Build history of the part. All positions in model axes, mm. A direction names the side the tool comes from. Give positions to 0.01 mm unless a question says otherwise; leave off trailing zeros. Order: outer loops, then holes, each group sorted by start corner. A loop starts at its lowest first (then second) coordinate and runs counter-clockwise, first axis right, second up. Notation, with made-up numbers: (1, -25.5) - (44, -25.5) arc R17 ccw to (44, -18.5) - close; hole circle Ø2 at (36.25, 11). An arc over 180 degrees is marked (long way). Use a Markdown table: item, result. Add a question column.
(1) Flat gauge pins, fed straight in: pin 1 (8 mm diameter, centred on x = 4, z = -31.5, fed in from -Y); pin 2 (8 mm diameter, centred on y = 38, z = 5.5, fed in from +X); pin 3 (5 mm diameter, centred on x = 7, y = 14, fed in from +Z). Where does each tip first touch, or does it go through?
(2) Mould opens along Z. For faces 5 (the face through (0, 39, 19)), 6 (the face through (-0.13, 35.9, 10.98)), 7 (the face through (0, 37, -198)), 8 (the face through (9, 41, 7)) say: +Z half, -Z half, draft (parallel to the pull), parting line (faces both ways), or undercut.
(3) Slice it at A-A (z = -42). Write the cut outline in (x, y).
(4) Slice it at D-D (x = -13.5). Write the cut outline in (y, z).
(5) Slice it at C-C (y = 14.5). Write the cut outline in (x, z), then the cut area to 3 significant figures.
(6) Slice it at B-B (z = 2). Write the cut outline in (x, y).
(7) Wall check: line 1 (Z direction, x = 0, y = 39); line 2 (Y direction, x = 0, z = -66.5); line 3 (Z direction, x = -6, y = 36). Give the ranges that are in metal, low to high.
(8) Which spindle directions (+Z, -Z, +X, -X, +Y, -Y) get a long thin tool onto all of the face, cutting with end or side? Do faces 1 (the face through (-9.237, 32.63, -188.367)), 2 (the face through (-13.047, 50.472, -97.88)), 3 (the face through (-7.797, 31.141, 9.633)), 4 (the face through (0, 48, 9)). Say none if no direction does.
from build123d import *

# Parameters (mm, degrees)
SKETCH_1_R               = 20
EXTRUDE_1_DEPTH          = 19
SKETCH_2_R               = 17
SKETCH_2_R_2             = 10
EXTRUDE_2_DEPTH          = 160
EXTRUDE_START            = 160
SKETCH_2_3_R             = 10
EXTRUDE_3_DEPTH          = 19
CUT_EXTRUDE_1_DEPTH      = 208.569265548
CUT_EXTRUDE_1_DEPTH_BACK = 208.569265548
SKETCH_3_R               = 3.25
SKETCH_4_R               = 19
EXTRUDE_4_DEPTH          = 75
SKETCH_5_W               = 18
SKETCH_5_H               = 18
EXTRUDE_5_DEPTH          = 19
FILLET_1_R               = 4
SKETCH_6_R               = 3.25
CUT_EXTRUDE_2_DEPTH      = 209.628857159


with BuildPart() as part:
    # Sketch 1 → Extrude 1 (new body)
    with BuildSketch(Plane.XY):
        with BuildLine():
            Line((-20, 49), (-20, 0))
            ThreePointArc((-20, 0), (0, 20), (20, 0))
            Line((20, 0), (20, 49))
            Line((20, 49), (10, 59))
            Line((10, 59), (-10, 59))
            Line((-10, 59), (-20, 49))
        make_face()
        Circle(SKETCH_1_R)
    extrude(amount=-EXTRUDE_1_DEPTH)

    # Sketch 2 → Extrude 2 (add)
    # profile 1 of 3: a face of its own
    with BuildSketch(Plane(origin=(0, 0, -19), x_dir=(-1, 0, 0), z_dir=(0, 0, -1))):
        with BuildLine():
            Line((10, 59), (-10, 59))
            Line((-10, 59), (-16.009113575, 42.179115539))
            ThreePointArc((-16.009113575, 42.179115539), (0, 53.46), (16.009113575, 42.179115539))
            Line((16.009113575, 42.179115539), (10, 59))
        make_face()
    # profile 2 of 3: a face of its own
    with BuildSketch(Plane(origin=(0, 0, -19), x_dir=(-1, 0, 0), z_dir=(0, 0, -1))):
        with Locations((0, 36.46)):
            Circle(SKETCH_2_R)
        with Locations((0, 36.46)):
            Circle(SKETCH_2_R_2, mode=Mode.SUBTRACT)
    # profile 3 of 3: a face of its own
    with BuildSketch(Plane(origin=(0, 0, -19), x_dir=(-1, 0, 0), z_dir=(0, 0, -1))):
        with Locations((0, 36.46)):
            Circle(SKETCH_2_R_2)
    extrude(amount=EXTRUDE_2_DEPTH)

    # Sketch 2_3 → Extrude 3 (add)
    with BuildSketch(Plane(origin=(0, 0, -19), x_dir=(-1, 0, 0), z_dir=(0, 0, -1)).offset(EXTRUDE_START)):
        with Locations((0, 36.46)):
            Circle(SKETCH_2_3_R)
    extrude(amount=EXTRUDE_3_DEPTH)

    # Sketch 3 → Cut-Extrude 1 (cut, two sides: drawn at the far end of the back side and taken through both)
    with BuildSketch(Plane(origin=(0, 0, 0), x_dir=(0, 0, -1), z_dir=(1, 0, 0)).offset(-CUT_EXTRUDE_1_DEPTH_BACK)):
        with Locations((189, 36)):
            Circle(SKETCH_3_R)
    extrude(amount=CUT_EXTRUDE_1_DEPTH + CUT_EXTRUDE_1_DEPTH_BACK, mode=Mode.SUBTRACT)

    # Sketch 4 → Extrude 4 (add)
    with BuildSketch(Plane(origin=(0, 0, -19), x_dir=(-1, 0, 0), z_dir=(0, 0, -1))):
        with Locations(Location((0, 0, 0), (0, 0, 180))):
            Circle(SKETCH_4_R)
    extrude(amount=EXTRUDE_4_DEPTH)

    # Sketch 5 → Extrude 5 (add)
    with BuildSketch(Plane.XY):
        with Locations((0, 39)):
            Rectangle(SKETCH_5_W, SKETCH_5_H)
    extrude(amount=EXTRUDE_5_DEPTH)

    # Fillet 1
    fillet_1_edges = [part.edges().sort_by_distance(p)[0] for p in [
        (9, 30, 9.5),
        (9, 48, 9.5),
        (-9, 48, 9.5),
        (-9, 30, 9.5),
    ]]
    fillet(fillet_1_edges, radius=FILLET_1_R)

    # Sketch 6 → Cut-Extrude 2 (cut, through all)
    with BuildSketch(Plane.ZY.offset(9)):
        with Locations(Location((10, 39, 0), (0, 0, 270))):
            Circle(SKETCH_6_R)
    extrude(amount=-CUT_EXTRUDE_2_DEPTH, mode=Mode.SUBTRACT)


solid = part.part
Solution:
| question | item | result |
|---|---|---|
| 1 | pin 1 | y = -19 |
| 1 | pin 2 | x = 9 |
| 1 | pin 3 | z = 0 |
| 2 | face 5 | +Z half |
| 2 | face 6 | undercut |
| 2 | face 7 | -Z half |
| 2 | face 8 | draft |
| 3 | outline | circle Ø38 at (0, 0); (-16.01, 42.18) arc R17 ccw (long way) to (16.01, 42.18) - (10, 59) - (-10, 59) - close |
| 4 | outline | (-14.76, -19) - (-13.37, -19) - (-13.37, -94) - (13.37, -94) - (13.37, -19) - (26.13, -19) - (26.13, -179) - (49.2, -179) - (49.2, -19) - (55.5, -19) - (55.5, 0) - (-14.76, 0) - close |
| 5 | outline | (-20, -19) - (-12.28, -19) - (-12.28, -94) - (12.28, -94) - (12.28, -19) - (20, -19) - (20, 0) - (-20, 0) - close |
| 5 | area | 2,600 mm2 |
| 6 | outline | (-9, 34) arc R4 ccw to (-5, 30) - (5, 30) arc R4 ccw to (9, 34) - (9, 44) arc R4 ccw to (5, 48) - (-5, 48) arc R4 ccw to (-9, 44) - close |
| 7 | line 1 | -198 to -190.25, -187.75 to 6.75, 13.25 to 19 |
| 7 | line 2 | -19 to 19, 19.46 to 59 |
| 7 | line 3 | -198 to -192.25, -185.75 to 8.75, 11.25 to 19 |
| 8 | face 1 | -Z |
| 8 | face 2 | -Z, -X, +Y |
| 8 | face 3 | +Z, -X, -Y |
| 8 | face 4 | +Z, +X, -X, +Y |
